from build123d import *

# Parameters (mm, degrees)
SKETCH1_W                 = 25
SKETCH1_H                 = 38
BOSS_EXTRUDE1_DEPTH       = 12
SKETCH3_W                 = 25
SKETCH3_H                 = 12
BOSS_EXTRUDE2_DEPTH       = 5.5
SKETCH5_W                 = 25
SKETCH5_H                 = 5
BOSS_EXTRUDE3_DEPTH       = 21
SKETCH6_R                 = 1.25
CUT_EXTRUDE1_DEPTH        = 10
SKETCH7_W                 = 210
SKETCH7_H                 = 85.25
BOSS_EXTRUDE4_DEPTH       = 5
SKETCH8_W                 = 10
SKETCH8_H                 = 60.2
BOSS_EXTRUDE5_DEPTH       = 210
CUT_EXTRUDE3_DEPTH        = 211
BOSS_EXTRUDE6_DEPTH       = 5
SKETCH11_W                = 10
SKETCH11_H                = 85.25
BOSS_EXTRUDE7_DEPTH       = 3.05
SKETCH12_W                = 10
SKETCH12_H                = 50
BOSS_EXTRUDE8_DEPTH       = 10.45
SKETCH13_W                = 70
SKETCH13_H                = 25
BOSS_EXTRUDE9_DEPTH       = 5
SKETCH14_W                = 68
SKETCH14_H                = 25
BOSS_EXTRUDE10_DEPTH      = 1.95
BOSS_EXTRUDE10_DEPTH_BACK = 3.05
SKETCH18_W                = 95.25
SKETCH18_H                = 60.2
CUT_EXTRUDE5_DEPTH        = 70
SKETCH19_W                = 68
SKETCH19_H                = 40
CUT_EXTRUDE6_DEPTH        = 94.2
SKETCH20_R                = 1.3890625
CUT_EXTRUDE7_DEPTH        = 10


with BuildPart() as part:
    # Sketch1 → Boss-Extrude1 (new body)
    with BuildSketch(Plane(origin=(0, 0, 0), x_dir=(1, 0, 0), z_dir=(0, 1, 0))):
        with Locations((12.5, 19)):
            Rectangle(SKETCH1_W, SKETCH1_H)
    extrude(amount=BOSS_EXTRUDE1_DEPTH)

    # Sketch3 → Boss-Extrude2 (add)
    with BuildSketch(Plane.XY):
        with Locations((12.5, 6)):
            Rectangle(SKETCH3_W, SKETCH3_H)
    boss_extrude2 = extrude(amount=BOSS_EXTRUDE2_DEPTH)

    # Sketch5 → Boss-Extrude3 (add)
    with BuildSketch(Plane.XZ):
        with Locations((12.5, 3)):
            Rectangle(SKETCH5_W, SKETCH5_H)
    boss_extrude3 = extrude(amount=BOSS_EXTRUDE3_DEPTH)

    # Sketch6 → Cut-Extrude1 (cut)
    with BuildSketch(Plane.XY.offset(5.5)):
        with Locations((3, -16.5)):
            Circle(SKETCH6_R)
        with Locations((22.59, -16.5)):
            Circle(SKETCH6_R)
        with Locations((22.59, -3.53)):
            Circle(SKETCH6_R)
        with Locations((3, -3.53)):
            Circle(SKETCH6_R)
    cut_extrude1 = extrude(amount=-CUT_EXTRUDE1_DEPTH, mode=Mode.SUBTRACT)

    # Mirror1: Boss-Extrude2, Boss-Extrude3, Cut-Extrude1 across plane
    add(boss_extrude2.mirror(Plane.XY.offset(-19)))
    add(boss_extrude3.mirror(Plane.XY.offset(-19)))
    add(cut_extrude1.mirror(Plane.XY.offset(-19)), mode=Mode.SUBTRACT)

    # Sketch7 → Boss-Extrude4 (add)
    with BuildSketch(Plane(origin=(0, 12, 0), x_dir=(1, 0, 0), z_dir=(0, 1, 0))):
        with Locations((12.5, 31.375)):
            Rectangle(SKETCH7_W, SKETCH7_H)
    extrude(amount=BOSS_EXTRUDE4_DEPTH)

    # Sketch8 → Boss-Extrude5 (add, through all)
    with BuildSketch(Plane(origin=(117.5, 0, 0), x_dir=(0, 0, -1), z_dir=(1, 0, 0))):
        with Locations((79, 42.1)):
            Rectangle(SKETCH8_W, SKETCH8_H)
    extrude(amount=-BOSS_EXTRUDE5_DEPTH)

    # Sketch9 → Cut-Extrude3 (cut, through all)
    with BuildSketch(Plane.ZY.offset(92.5)):
        Polygon((-74, 43.24), (-77.2, 41.128), (-77.2, 72.2), (-74, 72.2), align=None)
    extrude(amount=-CUT_EXTRUDE3_DEPTH, mode=Mode.SUBTRACT)

    # Sketch10 → Boss-Extrude6 (add)
    with BuildSketch(Plane(origin=(117.5, 0, 0), x_dir=(0, 0, -1), z_dir=(1, 0, 0))):
        Polygon((77.2, 72.2), (74, 72.2), (74, 43.24), (77.2, 41.128), align=None)
    extrude(amount=-BOSS_EXTRUDE6_DEPTH)

    # Sketch11 → Boss-Extrude7 (add)
    with BuildSketch(Plane(origin=(0, 17, 0), x_dir=(1, 0, 0), z_dir=(0, 1, 0))):
        with Locations((40.5, 31.375)):
            Rectangle(SKETCH11_W, SKETCH11_H)
        with Locations((-17.5, 31.375)):
            Rectangle(SKETCH11_W, SKETCH11_H)
    extrude(amount=BOSS_EXTRUDE7_DEPTH)

    # Sketch12 → Boss-Extrude8 (add)
    with BuildSketch(Plane(origin=(0, 17, 0), x_dir=(1, 0, 0), z_dir=(0, 1, 0))):
        with Locations((-87.5, 31.375)):
            Rectangle(SKETCH12_W, SKETCH12_H)
        with Locations((-37.5, 31.375)):
            Rectangle(SKETCH12_W, SKETCH12_H)
    extrude(amount=BOSS_EXTRUDE8_DEPTH)

    # Sketch13 → Boss-Extrude9 (add)
    with BuildSketch(Plane.XY.offset(11.25)):
        with Locations((82.5, 24.5)):
            Rectangle(SKETCH13_W, SKETCH13_H)
    extrude(amount=BOSS_EXTRUDE9_DEPTH)

    # Sketch14 → Boss-Extrude10 (add, two sides)
    with BuildSketch(Plane.XY.offset(11.25)) as boss_extrude10_sk:
        with Locations((11.5, 24.5)):
            Rectangle(SKETCH14_W, SKETCH14_H)
    extrude(amount=BOSS_EXTRUDE10_DEPTH)
    extrude(boss_extrude10_sk.sketch, amount=-BOSS_EXTRUDE10_DEPTH_BACK)

    # Sketch18 → Cut-Extrude5 (cut)
    with BuildSketch(Plane.ZY.offset(92.5)):
        with Locations((-36.375, 42.1)):
            Rectangle(SKETCH18_W, SKETCH18_H)
    extrude(amount=-CUT_EXTRUDE5_DEPTH, mode=Mode.SUBTRACT)

    # Sketch19 → Cut-Extrude6 (cut, through all)
    with BuildSketch(Plane(origin=(0, 72.2, 0), x_dir=(1, 0, 0), z_dir=(0, 1, 0))):
        with Locations((11.5, 64)):
            Rectangle(SKETCH19_W, SKETCH19_H)
    extrude(amount=-CUT_EXTRUDE6_DEPTH, mode=Mode.SUBTRACT)

    # Sketch20 → Cut-Extrude7 (cut)
    with BuildSketch(Plane(origin=(0, 72.2, 0), x_dir=(1, 0, 0), z_dir=(0, 1, 0))):
        with Locations((65.5, 80.6)):
            Circle(SKETCH20_R)
        with Locations((97.5, 80.6)):
            Circle(SKETCH20_R)
    extrude(amount=-CUT_EXTRUDE7_DEPTH, mode=Mode.SUBTRACT)


solid = part.part
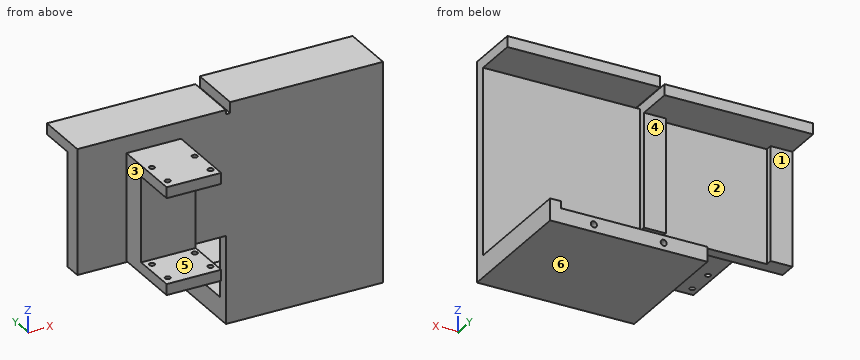
Here's how the part is built. I have some questions about the finished solid (model axes, mm). Face numbers are marked on the shaded views. A direction names the side the tool comes from. Give positions to 0.01 mm unless a question says otherwise; leave off trailing zeros. Write each loop counter-clockwise with the first axis right and the second up, starting at its lowest first coordinate (ties: lowest second). Pieces come first, ordered by that corner, then holes. Notation, with made-up numbers: (66, 2.25) -> (89, 2.25) arc R28 ccw to (89, 25.25) -> close; hole circle Ø10 at (-13, 52.25). An arc over 180 degrees is marked (long way). Use one line per item in the form item = value. Start each with the question number.
1. Imagine slicing it at C-C on x = 72. List the corners of the cut face in (y, z) for me, plus the area to 3 significant figures.
2. If I drill on L1, parallel to X at y = -16.5, z = -40.05; L2, parallel to Z at x = 97.5, y = 68.5; L3, parallel to Y at x = 22.59, z = -40.2, over which ranges is the centre line in solid material (lowest first)?
3. Imagine slicing it at D-D on z = -18.5. List the corners of the cut face in (x, y) for me.
4. Imagine slicing it at B-B on y = -7. List the corners of the cut face in (x, z) for me.
5. Thinking about a two-plate mould opening in Z: for the marked faces 4, 5 and 6, which applies, +Z half, -Z half, draft (parallel to the pull), parting line (faces both ways), or undercut?
6. On a 3-axis mill with a long thin cutter (end or side, diameter ignored), from which of +Z, -Z, +X, -X, +Y, -Y can I reach the whole of each face in a straight line? I mean the marked faces 1, 2 and 3. Say none if no direction works.
7. Imagine slicing it at A-A on y = 28.5. List the corners of the cut face in (x, z) for me.
8. Will these pins go through, and if not, where does the flat tip stop? pin 1 Ø8 at (x, z) = (39.5, -7.5) entering from +Y; pin 2 Ø3 at (x, z) = (62, 4) entering from +Y; pin 3 Ø23 at (x, y) = (16, -15.5) entering from -Z.
Entries:
q1.outline = (12, -84) -> (72.2, -84) -> (72.2, -77.2) -> (41.13, -77.2) -> (43.24, -74) -> (17, -74) -> (17, 11.25) -> (37, 11.25) -> (37, 16.25) -> (12, 16.25) -> close
q1.area = 1,060 mm²
q2.L1 = 0 to 1.75, 4.25 to 21.34, 23.84 to 25
q2.L2 = -84 to -81.99, -79.21 to -77.2
q2.L3 = -21 to -17.75, -15.25 to -4.78, -2.28 to 17
q3.outline = (-22.5, 12) -> (0, 12) -> (0, 0) -> (25, 0) -> (25, 12) -> (117.5, 12) -> (117.5, 17) -> (45.5, 17) -> (45.5, 20.05) -> (35.5, 20.05) -> (35.5, 17) -> (-12.5, 17) -> (-12.5, 20.05) -> (-22.5, 20.05) -> close
q4.outline = (0, -43.5) -> (25, -43.5) -> (25, -38.5) -> (0, -38.5) -> close; (0, 0.5) -> (25, 0.5) -> (25, 5.5) -> (0, 5.5) -> close
q5.face_4 = draft
q5.face_5 = undercut
q5.face_6 = -Z half
q6.face_1 = -Z, +X, -X, +Y
q6.face_2 = -Z, +Y
q6.face_3 = +Z, -Z, -X, -Y
q7.outline = (-22.5, 8.2) -> (45.5, 8.2) -> (45.5, 13.2) -> (-22.5, 13.2) -> close; (45.5, -84) -> (117.5, -84) -> (117.5, -74) -> (45.5, -74) -> close; (47.5, 11.25) -> (117.5, 11.25) -> (117.5, 16.25) -> (47.5, 16.25) -> close
q8.pin_1 = 20.05
q8.pin_2 = 17
q8.pin_3 = -43.5
